```python
from build123d import *

# Parameters (mm, degrees)
F0_W        = 101.6
F0_H        = 25.4
F1_DEPTH    = 25.4
F2_W        = 25.4
F2_H        = 25.4
F3_DEPTH    = 25.4
F4_W        = 76.2
F4_H        = 25.4
F4_W_2      = 25.4
F5_DEPTH    = 25.4
F6_W        = 25.4
F6_H        = 25.4
F7_DEPTH    = 156.21
F8_T1_DEPTH = 286.6829915773
F8_T3_DEPTH = 286.6829915773


# Not quite as in the source:
# - a fillet or chamfer that OpenCascade refuses, or shapes differently, is made with other operations: its cross-section is extruded or revolved along the edge and cut away or added


with BuildPart() as f1:
    # F0 (on Right) → F1 (new body)
    with BuildSketch(Plane.YZ):
        Rectangle(F0_W, F0_H)
    extrude(amount=F1_DEPTH)

    # F2 (on face) → F3 (join)
    with BuildSketch(Plane.YZ.offset(25.4)):
        with Locations((38.1, 0)):
            Rectangle(F2_W, F2_H)
        with Locations((-38.1, 0)):
            Rectangle(F2_W, F2_H)
    extrude(amount=F3_DEPTH)

    # F4 (on face) → F5 (join)
    with BuildSketch(Plane.YZ.offset(50.8)):
        with Locations((12.7, 0)):
            Rectangle(F4_W, F4_H)
        with Locations((-38.1, 0)):
            Rectangle(F4_W_2, F4_H)
    extrude(amount=F5_DEPTH)

    # F6 (on face) → F7 (join)
    with BuildSketch(Plane(origin=(0, 0, -12.7), x_dir=(1, 0, 0), z_dir=(0, 0, -1))):
        with Locations((63.5, 38.1)):
            Rectangle(F6_W, F6_H)
        with Locations((63.5, -38.1)):
            Rectangle(F6_W, F6_H)
    extrude(amount=F7_DEPTH)

    # F8: chamfer of 50.8 on 2 edges, made by hand

    # F8_s2 → F8_t1 (cut)
    with BuildSketch(Plane.XZ.offset(-181.4414957887)):
        Polygon((76.2, -118.11), (25.4, -168.91), (76.2, -168.91), align=None)
    extrude(amount=F8_T1_DEPTH, mode=Mode.SUBTRACT)

    # F8_s4 → F8_t3 (cut)
    with BuildSketch(Plane.XZ.offset(-105.2414957887)):
        Polygon((25.4, -168.91), (76.2, -118.11), (76.2, -168.91), align=None)
    extrude(amount=F8_T3_DEPTH, mode=Mode.SUBTRACT)


solid = f1.part
```
Build history of the part. All positions in model axes, mm. A direction names the side the tool comes from. Coordinates: 2 decimals unless noted, no trailing zeros. Write each loop counter-clockwise with the first axis right and the second up, starting at its lowest first coordinate (ties: lowest second). Pieces come first, ordered by that corner, then holes.
1. Band-saw the part on D-D, the plane x = 63.5. Give the cut face in (y, z).
Answer block:
outline: (-50.8, -130.81) - (-25.4, -130.81) - (-25.4, -12.7) - (25.4, -12.7) - (25.4, -130.81) - (50.8, -130.81) - (50.8, 12.7) - (-50.8, 12.7) - close
2. Band-saw the part on C-C, the plane z = -8.5. Give the cut face in (x, y), and give its area (3 significant figures).
Answer block:
outline: (0, -50.8) - (76.2, -50.8) - (76.2, 50.8) - (0, 50.8) - close; hole (25.4, -25.4) - (50.8, -25.4) - (50.8, 25.4) - (25.4, 25.4) - close
area: 6,450 mm2
3. 3-axis set-ups, long thin cutter, end or side, ignore diameter. For faces 1 (the flat face through (63.68, -37.92, -130.63)), 2 (the flat face through (63, -25.4, -77)), 3 (the flat face through (50.8, 38, -77)), 4 (the flat face through (50.8, 0, 0)): which of +Z, -Z, +X, -X, +Y, -Y reach the whole face in a straight line?
Answer block:
face 1: -Z, +X, +Y, -Y
face 2: -Z, +X, -X
face 3: -Z, -X, +Y, -Y
face 4: +Z, -Z
4. Band-saw the part on A-A, the plane z = -132.5. Give the cut face in (x, y), and give its area (3 significant figures).
Answer block:
outline: (50.8, -50.8) - (61.81, -50.8) - (61.81, -25.4) - (50.8, -25.4) - close; (50.8, 25.4) - (61.81, 25.4) - (61.81, 50.8) - (50.8, 50.8) - close
area: 559 mm2
5. Drill centre lines: probe 1 along Y at (x, z) = (60.5, -85.5); probe 2 along X at (y, z) = (19.5, 2.5); probe 3 along X at (y, z) = (-38, -25). Where is each one in solid material? Low to high.
Answer block:
probe 1: y = -50.8 to -25.4, 25.4 to 50.8
probe 2: x = 0 to 25.4, 50.8 to 76.2
probe 3: x = 50.8 to 76.2
6. Drop flat-ended pins along their axis: pin 1 (2 mm diameter, centred on y = 28.5, z = -30.5, fed in from -X); pin 2 (1.5 mm diameter, centred on x = 10.5, y = -15, fed in from -Z); pin 3 (2 mm diameter, centred on x = 27.5, y = 8.5, fed in from +Z); pin 4 (12.5 mm diameter, centred on y = -1, z = -5.5, fed in from -X). Give the stop position or say it passes through.
Answer block:
pin 1: stops at x = 50.8
pin 2: stops at z = -12.7
pin 3: passes through
pin 4: stops at x = 0
7. Pull direction X, two halves, no side cores. Call faces 5 (the flat face through (54, 1, 12.7)), 6 (the flat face through (76.2, 1, -8)), 7 (the flat face through (38, -25.4, 0)), 8 (the flat face through (25.4, 0, 0)): released by +X, released by -X, zero draft, split by the parting line, or undercut.
Answer block:
face 5: zero draft
face 6: released by +X
face 7: undercut
face 8: undercut
8. Band-saw the part on B-B, the plane x = 38.5. Give the cut face in (y, z), and give its area (3 significant figures).
Answer block:
outline: (-50.8, -12.7) - (-25.4, -12.7) - (-25.4, 12.7) - (-50.8, 12.7) - close; (25.4, -12.7) - (50.8, -12.7) - (50.8, 12.7) - (25.4, 12.7) - close
area: 1,290 mm2
